Could you check a few things on this model? Use its own coordinates, in mm. A direction names the side the tool comes from. Give positions to 0.01 mm unless a question says otherwise; leave off trailing zeros. Write each loop counter-clockwise with the first axis right and the second up, starting at its lowest first coordinate (ties: lowest second). Pieces come first, ordered by that corner, then holes. Notation, with made-up numbers: M 40,84.25 L 71,84.25 A22 ccw 71,92.25 Z; hole C 15,31 d5. An arc over 180 degrees is marked long. Use one line per item in the form item = value.
from build123d import *

# Parameters (mm, degrees)
SKETCH1_W           = 636
SKETCH1_H           = 800
BOSS_EXTRUDE1_DEPTH = 18
BOSS_EXTRUDE2_DEPTH = 636
SKETCH4_W           = 636
SKETCH4_H           = 18
BOSS_EXTRUDE3_DEPTH = 1084
SKETCH5_W           = 636
SKETCH5_H           = 800
BOSS_EXTRUDE4_DEPTH = 18
BOSS_EXTRUDE6_DEPTH = 18
SKETCH11_W          = 18
SKETCH11_H          = 800
BOSS_EXTRUDE7_DEPTH = 1084
SKETCH13_W          = 636
SKETCH13_H          = 18
SKETCH15_W          = 18
SKETCH15_H          = 800
BOSS_EXTRUDE8_DEPTH = 1084
SKETCH16_R          = 228.5
CUT_EXTRUDE1_DEPTH  = 18.1
SKETCH17_W          = 18
SKETCH17_H          = 18
BOSS_EXTRUDE9_DEPTH = 18


with BuildPart() as part:
    # Sketch1 → Boss-Extrude1 (new body)
    with BuildSketch(Plane(origin=(0, 0, 0), x_dir=(1, 0, 0), z_dir=(0, 1, 0))):
        Rectangle(SKETCH1_W, SKETCH1_H)
    extrude(amount=BOSS_EXTRUDE1_DEPTH)

    # Sketch3 → Boss-Extrude2 (add)
    with BuildSketch(Plane.ZY.offset(318)):
        Polygon((139.336620479, 18), (228, 18), (228, 19.102485389), (-15, 66.336900509), (-219, 199.336900509), (-339.866628021, 382), (-382, 613.733545883), (-382, 547), (-352, 382), (-219, 181), (-15, 48), align=None)
        Polygon((360, 602), (360, 1102), (342, 1102), (342, 616.063141277), (24.044559613, 536.787946332), (-78.801457937, 659.355057231), (-101.379606002, 874.171786631), (-119.281000119, 872.290274292), (-96.127616004, 652.00053947), (4.612607271, 531.943016464), (17.485608625, 516.601570853), (342, 597.512095949), align=None)
        Polygon((112, 682), (112, 1102), (94, 1102), (94, 995.153242294), (2.678735209, 1102), (-21, 1102), (94, 967.448894468), (94, 682), align=None)
        Polygon((-226, 1102), (-253.559600781, 1102), (-382, 991.219245449), (-382, 967.448894468), align=None)
    extrude(amount=-BOSS_EXTRUDE2_DEPTH)


with BuildPart() as boss_extrude2_piece_1:
    # of the separate pieces the step leaves, piece 1, a body of its own (boss_extrude2_pieces)
    add(part.part.solids().sort_by_distance((-318, 0, 400))[0])



with BuildPart() as boss_extrude2_piece_2:
    # of the separate pieces the step leaves, piece 2, a body of its own (boss_extrude2_pieces)
    add(part.part.solids().sort_by_distance((-318, 602, 360))[0])


with BuildPart() as boss_extrude2_piece_3:
    # of the separate pieces the step leaves, piece 3, a body of its own (boss_extrude2_pieces)
    add(part.part.solids().sort_by_distance((-318, 682, 112))[0])


with BuildPart() as boss_extrude2_piece_4:
    # of the separate pieces the step leaves, piece 4, a body of its own (boss_extrude2_pieces)
    add(part.part.solids().sort_by_distance((-318, 1102, -226))[0])


with BuildPart() as boss_extrude2_piece_1_1:
    add(boss_extrude2_piece_1.part)

    add(boss_extrude2_piece_4.part)  # Boss-Extrude3 merges Boss-Extrude2 piece 4
    # Sketch4 → Boss-Extrude3 (add)
    with BuildSketch(Plane(origin=(0, 18, 0), x_dir=(1, 0, 0), z_dir=(0, 1, 0))):
        with Locations((0, 391)):
            Rectangle(SKETCH4_W, SKETCH4_H)
    extrude(amount=BOSS_EXTRUDE3_DEPTH)


    add(boss_extrude2_piece_2.part)  # Boss-Extrude4 merges Boss-Extrude2 piece 2

    add(boss_extrude2_piece_3.part)  # Boss-Extrude4 merges Boss-Extrude2 piece 3
    # Sketch5 → Boss-Extrude4 (add)
    with BuildSketch(Plane(origin=(0, 1102, 0), x_dir=(1, 0, 0), z_dir=(0, 1, 0))):
        Rectangle(SKETCH5_W, SKETCH5_H)
    extrude(amount=BOSS_EXTRUDE4_DEPTH)

    # Sketch10 → Boss-Extrude6 (add)
    with BuildSketch(Plane.ZY.offset(9)):
        Polygon((400, 18), (228, 18), (228, 569.088703625), (360, 602), (400, 602), align=None)
    extrude(amount=-BOSS_EXTRUDE6_DEPTH)

    # Sketch11 → Boss-Extrude7 (add)
    with BuildSketch(Plane(origin=(0, 18, 0), x_dir=(1, 0, 0), z_dir=(0, 1, 0))):
        with Locations((309, 0)):
            Rectangle(SKETCH11_W, SKETCH11_H)
    extrude(amount=BOSS_EXTRUDE7_DEPTH)

    # Sweep1: sweep along a path in Sketch14
    with BuildLine(Plane.ZY.offset(9)) as sweep1_path:
        Line((228, 261), (400, 301))
    # Sketch13 → Sweep1 (sweep)
    with BuildSketch(Plane(origin=(0, 0, 228), x_dir=(-1, 0, 0), z_dir=(0, 0, -1))):
        with Locations((0, 270)):
            Rectangle(SKETCH13_W, SKETCH13_H)
    sweep(path=sweep1_path.line)

    # Sketch15 → Boss-Extrude8 (add)
    with BuildSketch(Plane(origin=(0, 18, 0), x_dir=(1, 0, 0), z_dir=(0, 1, 0))):
        with Locations((-309, 0)):
            Rectangle(SKETCH15_W, SKETCH15_H)
    extrude(amount=BOSS_EXTRUDE8_DEPTH)

    # Sketch16 → Cut-Extrude1 (cut)
    with BuildSketch(Plane.XY.offset(360)):
        with Locations((0, 852)):
            Circle(SKETCH16_R)
    extrude(amount=-CUT_EXTRUDE1_DEPTH, mode=Mode.SUBTRACT)

    # Sketch17 → Boss-Extrude9 (add)
    with BuildSketch(Plane.XY.offset(360)):
        Polygon((300, 1102), (107, 1102), (125, 1084), (282, 1084), (282, 620), (300, 620), align=None)
        Polygon((-282, 620), (-282, 1084), (-125, 1084), (-107, 1102), (-300, 1102), (-300, 1084), (-300, 602), (-107, 602), (-125, 620), align=None)
        with Locations((291, 611)):
            Rectangle(SKETCH17_W, SKETCH17_H)
        Polygon((282, 602), (282, 620), (125, 620), (107, 602), align=None)
    extrude(amount=BOSS_EXTRUDE9_DEPTH)


solid = boss_extrude2_piece_1_1.part
1) I want a section at A-A, the plane y = 95. Please give me the cut outline in (x, z), plus the area to 3 significant figures.
Checked values:
outline = M -318,-400 L 318,-400 L 318,400 L 300,400 L 300,-58.96 L -300,-58.96 L -300,400 L -318,400 Z; M -9,228 L 9,228 L 9,400 L -9,400 Z; hole M -300,-382 L 300,-382 L 300,-87.09 L -300,-87.09 Z
area = 59,600 mm2
2) If I drill on L1, parallel to X at y = 123.5, z = 324; L2, parallel to X at y = 584, z = -142; L3, parallel to Z at x = 41, y = 768, over which ranges is the centre line in solid material (lowest first)?
Checked values:
L1 = -318 to -300, -9 to 9, 300 to 318
L2 = -318 to -300, 300 to 318
L3 = -400 to -382, -108.32 to -90.22, 94 to 112
3) Thinking about a two-plate mould opening in Y: for faces 4 (the flat face through (-4, 1102, 384)), 5 (the flat face through (-1, 474, 400)), which applies, released by +Y, released by -Y, zero draft, split by the parting line, or undercut?
Checked values:
face_4 = undercut
face_5 = zero draft
4) For faces 1 (the flat face through (-300, 552, 14)), 2 (the flat face through (-4, 552, -400)), 3 (the flat face through (9, 161, 315)), which set-ups out of +Z, -Z, +X, -X, +Y, -Y let a thin tool reach every point of the face, with its end or its side?
Checked values:
face_1 = none
face_2 = -Z, +X, -X, +Y, -Y
face_3 = +Z
5) For pin 1 Ø6 at (x, y) = (222.5, 607) entering from +Z; pin 2 Ø3 at (x, y) = (172, 394) entering from +Z, each with a flat end and sliding along its axis, tell me the tip position at first contact or that it passes through.
Checked values:
pin_1 = 378
pin_2 = -341.78
6) I want a section at B-B, the plane x = -244. Count the separate pieces of the cut face and the enclosed holes in it, plus the area to 4 significant figures.
Checked values:
separate_pieces = 2
enclosed_holes = 3
area = 100,000 mm2
7) I want a section at C-C, the plane y = 900. Please give me the cut outline in (x, z), plus the area to 3 significant figures.
Checked values:
outline = M -318,-400 L 318,-400 L 318,400 L 300,400 L 300,378 L 282,378 L 282,360 L 223.4,360 L 223.4,342 L 300,342 L 300,112 L -300,112 L -300,342 L -223.4,342 L -223.4,360 L -282,360 L -282,378 L -300,378 L -300,400 L -318,400 Z; hole M -300,-382 L 300,-382 L 300,94 L -300,94 Z
area = 53,800 mm2
